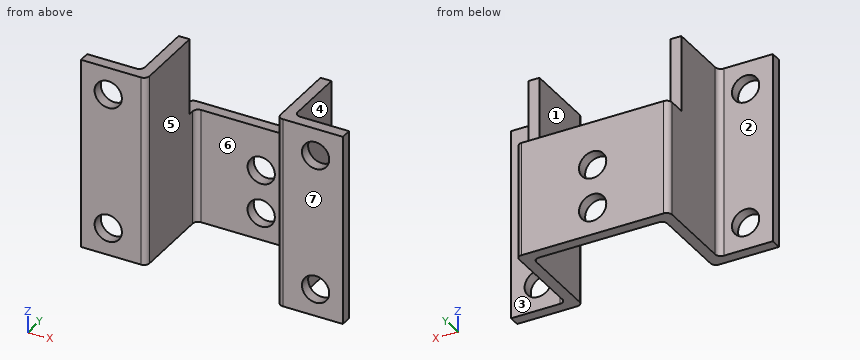
```python
from build123d import *

# Parameters (mm, degrees)
BOSS_EXTRUDE1_DEPTH     = 35
SKETCH2_W               = 14
SKETCH2_H               = 4
CUT_EXTRUDE1_DEPTH      = 55.083269132
CUT_EXTRUDE2_DEPTH      = 46.354161882
CUT_EXTRUDE2_DEPTH_BACK = 46.354161882
SKETCH3_R               = 2.5


with BuildPart() as part:
    # Sketch1 → Boss-Extrude1 (new body)
    with BuildSketch(Plane.XY):
        with BuildLine():
            Line((-24, 0), (-15, 0))
            ThreePointArc((-15, 0), (-14.292893219, 0.292893219), (-14, 1))
            Line((-14, 1), (-14, 15))
            ThreePointArc((-14, 15), (-13.707106781, 15.707106781), (-13, 16))
            Line((-13, 16), (13, 16))
            ThreePointArc((13, 16), (13.707106781, 15.707106781), (14, 15))
            Line((14, 15), (14, 1))
            ThreePointArc((14, 1), (14.292893219, 0.292893219), (15, 0))
            Line((15, 0), (24, 0))
            Line((24, 0), (24, -2))
            Line((24, -2), (13, -2))
            ThreePointArc((13, -2), (12.292893219, -1.707106781), (12, -1))
            Line((12, -1), (12, 13))
            ThreePointArc((12, 13), (11.707106781, 13.707106781), (11, 14))
            Line((11, 14), (-11, 14))
            ThreePointArc((-11, 14), (-11.707106781, 13.707106781), (-12, 13))
            Line((-12, 13), (-12, -1))
            ThreePointArc((-12, -1), (-12.292893219, -1.707106781), (-13, -2))
            Line((-13, -2), (-24, -2))
            Line((-24, -2), (-24, 0))
        make_face()
    extrude(amount=BOSS_EXTRUDE1_DEPTH)

    # Sketch2 → Cut-Extrude1 (cut, through all)
    with BuildSketch(Plane(origin=(14, 0, 0), x_dir=(0, 0, -1), z_dir=(1, 0, 0))):
        with Locations((-28, 14)):
            Rectangle(SKETCH2_W, SKETCH2_H)
    extrude(amount=-CUT_EXTRUDE1_DEPTH, mode=Mode.SUBTRACT)

    # Sketch3 → Cut-Extrude2 (cut, two sides: drawn at the far end of the back side and taken through both)
    with BuildSketch(Plane(origin=(0, 0, 0), x_dir=(1, 0, 0), z_dir=(0, 1, 0)).offset(-CUT_EXTRUDE2_DEPTH_BACK)):
        with Locations(Location((-19, -5, 0), (0, 0, 180))):
            Circle(SKETCH3_R)
        with Locations(Location((-19, -30, 0), (0, 0, 180))):
            Circle(SKETCH3_R)
        with Locations((19, -30)):
            Circle(SKETCH3_R)
        with Locations((19, -5)):
            Circle(SKETCH3_R)
        with Locations(Location((0, -13, 0), (0, 0, 180))):
            Circle(SKETCH3_R)
        with Locations(Location((0, -5, 0), (0, 0, 180))):
            Circle(SKETCH3_R)
    extrude(amount=CUT_EXTRUDE2_DEPTH + CUT_EXTRUDE2_DEPTH_BACK, mode=Mode.SUBTRACT)


solid = part.part
```
Input: part model. Units: mm. Frame: model coordinates. Face numbers are marked on the shaded views. A direction names the side the tool comes from. Round coordinates to 2 decimals unless told otherwise and drop trailing zeros. Order: outer loops, then holes, each group sorted by start corner. A loop starts at its lowest first (then second) coordinate and runs counter-clockwise, first axis right, second up. Notation, with made-up numbers: (-17, 15.5) - (-13, 15.5) arc R17 cw to (-13, 22.5) - close; hole circle Ø5 at (75.5, 4). An arc over 180 degrees is marked (long way). One line per question, with ' | ' between items. Start each with the question number.
1) Cut plane C-C, the plane x = 1.5. Return the cut outline in (y, z), then the cut area to 3 significant figures.
2) Ray query, probe 1 along Z at (x, y) = (-19, -0.95); probe 2 along Z at (x, y) = (0, 15.45); probe 3 along X at (y, z) = (4.25, 23). Return the intervals inside material, ascending.
3) Cut plane D-D, the plane z = 31.5. Return the cut outline in (x, y).
4) Contact query for flat-ended pins moving along their axis: P1, Ø1, axis at x = 5.5, z = 14.5, coming from the -Y side; P2, Ø3, axis at x = 2, y = 13, coming from the +Z side; P3, Ø4, axis at y = 4, z = 23.5, coming from the -X side. Output: stop coordinate, or through.
5) Cut plane B-B, the plane y = 7.5. Return the cut outline in (x, z).
6) Pull-direction query (X, two-part tool) for the marked faces 4, 5, 6 and 7; classes: +X half, -X half, draft (parallel to the pull), parting line (faces both ways), or undercut.
7) Set-up query: the marked faces 1, 2 and 3. Return all of +Z, -Z, +X, -X, +Y, -Y with unobstructed straight access to the full face (end or side cutting, diameter ignored); none if empty.
8) Cut plane A-A, the plane z = 26. Return the cut outline in (x, y), then the cut area to 3 significant figures.
Worked out:
1) outline: (14, 0) - (16, 0) - (16, 3) - (14, 3) - close; (14, 7) - (16, 7) - (16, 11) - (14, 11) - close; (14, 15) - (16, 15) - (16, 21) - (14, 21) - close | area: 26.0 mm^2
2) probe 1: z = 0 to 2.5, 7.5 to 27.5, 32.5 to 35 | probe 2: z = 0 to 2.5, 7.5 to 10.5, 15.5 to 21 | probe 3: x = -14 to -12, 12 to 14
3) outline: (-24, -2) - (-21, -2) - (-21, 0) - (-24, 0) - close; (-17, -2) - (-13, -2) arc R1 ccw to (-12, -1) - (-12, 12) - (-14, 12) - (-14, 1) arc R1 cw to (-15, 0) - (-17, 0) - close; (12, -1) arc R1 ccw to (13, -2) - (17, -2) - (17, 0) - (15, 0) arc R1 cw to (14, 1) - (14, 12) - (12, 12) - close; (21, -2) - (24, -2) - (24, 0) - (21, 0) - close
4) P1: stops at y = 14 | P2: stops at z = 21 | P3: stops at x = -14
5) outline: (-14, 0) - (-12, 0) - (-12, 35) - (-14, 35) - close; (12, 0) - (14, 0) - (14, 35) - (12, 35) - close
6) face 4: +X half | face 5: undercut | face 6: undercut | face 7: draft
7) face 1: +Z, -Z, -Y | face 2: +Z, -Z, -X, +Y | face 3: +Z, -Z, +X, +Y
8) outline: (-24, -2) - (-13, -2) arc R1 ccw to (-12, -1) - (-12, 12) - (-14, 12) - (-14, 1) arc R1 cw to (-15, 0) - (-24, 0) - close; (12, -1) arc R1 ccw to (13, -2) - (24, -2) - (24, 0) - (15, 0) arc R1 cw to (14, 1) - (14, 12) - (12, 12) - close | area: 96.0 mm^2
